```python
from build123d import *

# Parameters (mm, degrees)
CUT_EXTRUDE_1_DEPTH = 3


with BuildPart() as part:
    # Эскиз1 → Повернуть1 (revolve)
    with BuildSketch(Plane.XY):
        Polygon((0, 0), (3.2, 0), (4, 0.8), (4, 10), (0, 10), align=None)
    revolve(axis=Axis((0, 68.644575989, 0), (0, -1, 0)))

    # Эскиз2 → Вырез-Вытянуть1 (cut)
    with BuildSketch(Plane(origin=(0, 10, 0), x_dir=(1, 0, 0), z_dir=(0, 1, 0))):
        Polygon((1.755265403, -2.986476748), (3.463997433, 0.026866056), (1.708732029, 3.013342804), (-1.755265403, 2.986476748), (-3.463997433, -0.026866056), (-1.708732029, -3.013342804), align=None)
    extrude(amount=-CUT_EXTRUDE_1_DEPTH, mode=Mode.SUBTRACT)


solid = part.part
```
Work out the finished part from the listing and answer in its coordinate system (mm). A direction names the side the tool comes from. Coordinates: 2 decimals unless noted, no trailing zeros. Loops run counter-clockwise (first coordinate to the right, second up) from the corner with the lowest first, then second, coordinate; pieces in that order, holes last.
1) Flat-ended cylindrical pins translate along their axes: pin 1 (3 mm diameter, centred on y = 2, z = 2, fed in from -X); pin 2 (1.5 mm diameter, centred on x = 1, y = 7.5, fed in from +Z). Find the tip coordinate at first contact, or state that the pin passes through.
Results:
pin 1: stops at x = -3.97
pin 2: stops at z = 3.99
2) For a pull along Z with two mould halves and no side action, classify faces 3 (the flat face through (0, 7, 0)), 4 (the flat face through (-2.6, 8.5, -1.5)), 5 (the flat face through (0, 0, 0)), 6 (the cylindrical face through (-0.867, 5.464, -3.905)) as +Z half, -Z half, draft (parallel to the pull), parting line (faces both ways), or undercut.
Results:
face 3: undercut
face 4: undercut
face 5: draft
face 6: parting line
3) For faces 1 (the flat face through (2.6, 8.5, 1.5)), 2 (the flat face through (3, 10, 2)), determine the directions among +Z, -Z, +X, -X, +Y, -Y from which every point of the face is accessible in a straight line to the end or side of a thin tool.
Results:
face 1: +Y
face 2: +Z, -Z, +X, -X, +Y
4) Section C-C (y = 2.5) is taken. Give the vertices of the cut face in (x, z).
Results:
outline: circle Ø8 at (0, 0)
5) Consider probe 1 along Y at (x, z) = (-1.5, 1.5); probe 2 along Z at (x, y) = (1.5, 9.75); probe 3 along X at (y, z) = (8.75, 2.25). Determine where each line is inside the solid, lowest interval first.
Results:
probe 1: y = 0 to 7
probe 2: z = -3.71 to -3.01, 2.99 to 3.71
probe 3: x = -3.31 to -2.16, 2.17 to 3.31
6) Section A-A (y = 8) is taken. Give the vertices of the cut face in (x, z).
Results:
outline: circle Ø8 at (0, 0); hole (-3.46, 0.03) - (-1.76, -2.99) - (1.71, -3.01) - (3.46, -0.03) - (1.76, 2.99) - (-1.71, 3.01) - close
7) Section B-B (x = 0) is taken. Give the vertices of the cut face in (y, z).
Results:
outline: (0, -3.2) - (0.8, -4) - (10, -4) - (10, -3) - (7, -3) - (7, 3) - (10, 3) - (10, 4) - (0.8, 4) - (0, 3.2) - close
